```python
from build123d import *

# Parameters (mm, degrees)
F1_DEPTH  = 25
F2_W      = 2.8
F2_H      = 0.75
F3_DEPTH  = 1.5
F4_W      = 3.6
F4_H      = 1
F5_DEPTH  = 0.5
F6_W      = 10
F6_H      = 0.25
F7_DEPTH  = 0.2
F8_W      = 10
F8_H      = 14.625
F9_DEPTH  = 4.201
F10_R     = 1
F12_DEPTH = 2.701


with BuildPart() as f1:
    # F0 (on Front) → F1 (new body, symmetric)
    with BuildSketch(Plane.XZ):
        Polygon((-5, 4.2), (-5, 0), (5, 0), (5, 4.2), (1.4, 4.2), (1.4, 2), (-1.4, 2), (-1.4, 4.2), align=None)
    extrude(amount=F1_DEPTH, both=True)

    # F2 (on face) → F3 (join)
    with BuildSketch(Plane.XY.offset(2)):
        Rectangle(F2_W, F2_H)
    extrude(amount=F3_DEPTH)

    # F4 (on face) → F5 (join)
    with BuildSketch(Plane.XY.offset(4.2)):
        with Locations((3.2, -0.875)):
            Rectangle(F4_W, F4_H)
        with Locations((-3.2, -0.875)):
            Rectangle(F4_W, F4_H)
    extrude(amount=F5_DEPTH)

    # F6 (on face) → F7 (cut)
    with BuildSketch(Plane.XY.offset(4.2)):
        with Locations((0, -6.375)):
            Rectangle(F6_W, F6_H)
        with Locations((0, -11.375)):
            Rectangle(F6_W, F6_H)
        with Locations((0, -16.375)):
            Rectangle(F6_W, F6_H)
    extrude(amount=-F7_DEPTH, mode=Mode.SUBTRACT)

    # F8 (on face) → F9 (cut, through all)
    with BuildSketch(Plane.XY.offset(4.2)):
        with Locations((0, 17.6875)):
            Rectangle(F8_W, F8_H)
    extrude(amount=-F9_DEPTH, mode=Mode.SUBTRACT)

    # F10
    f10_edges = [f1.edges().sort_by_distance(p)[0] for p in [
        (-5, 10.375, 2.1),
        (5, 10.375, 2.1),
        (-5, -25, 2.1),
        (5, -25, 2.1),
    ]]
    fillet(f10_edges, radius=F10_R)

    # F11 (on face) → F12 (cut, through all)
    with BuildSketch(Plane.XY.offset(2)):
        Polygon((2, -0.375), (-2, -0.375), (-1.4, -3.375), (1.4, -3.375), align=None)
        Polygon((-1.4, 3.375), (-2, 0.375), (2, 0.375), (1.4, 3.375), align=None)
    extrude(amount=F12_DEPTH, mode=Mode.SUBTRACT)


solid = f1.part
```
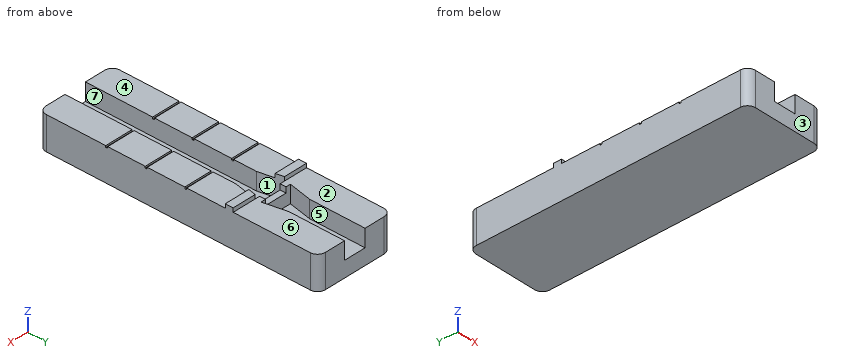
Read the model definition and answer for the solid it produces. Units are mm, in the model's axes. Face numbers are marked on the shaded views. A direction names the side the tool comes from. Coordinates: 2 decimals unless noted, no trailing zeros. Write each loop counter-clockwise with the first axis right and the second up, starting at its lowest first coordinate (ties: lowest second). Pieces come first, ordered by that corner, then holes. Notation, with made-up numbers: (-27.75, 20.25) -> (25.25, 20.25) arc R28 ccw to (25.25, 51.25) -> close; hole circle Ø1 at (56, 52.5). An arc over 180 degrees is marked (long way). Return JSON: item names as keys, results as strings.
1. Each of these flat-tipped pins is pushed along its axis until it touches: P1, Ø4, axis at x = 4, y = -4.5, coming from the +Z side; P2, Ø3, axis at x = -4, y = -2.5, coming from the +Z side. Where does it stop, or does it pass through?
Found:
{"P1": "z = 4.2", "P2": "z = 4.7"}
2. A cutting plane is placed at D-D (x = -2.75). Determine the outline of the cut face in (y, z) (3 decimals), and give its area (3 significant figures).
Found:
{"outline": "(-25, 0) -> (10.375, 0) -> (10.375, 4.2) -> (-0.375, 4.2) -> (-0.375, 4.7) -> (-1.375, 4.7) -> (-1.375, 4.2) -> (-6.25, 4.2) -> (-6.25, 4) -> (-6.5, 4) -> (-6.5, 4.2) -> (-11.25, 4.2) -> (-11.25, 4) -> (-11.5, 4) -> (-11.5, 4.2) -> (-16.25, 4.2) -> (-16.25, 4) -> (-16.5, 4) -> (-16.5, 4.2) -> (-25, 4.2) -> close", "area": "149 mm2"}
3. Find the intervals of material crossed by line 1 along X through (y, z) = (-22, 2.6); line 2 along Z through (x, y) = (-2.75, -23); line 3 along Z through (x, y) = (-1.25, -13), in increasing order. Write a range as from..to.
Found:
{"line 1": "-5..-1.4, 1.4..5", "line 2": "0..4.2", "line 3": "0..2"}
4. A cutting plane is placed at A-A (y = -15). Determine the outline of the cut face in (x, z), and give its area (3 significant figures).
Found:
{"outline": "(-5, 0) -> (5, 0) -> (5, 4.2) -> (1.4, 4.2) -> (1.4, 2) -> (-1.4, 2) -> (-1.4, 4.2) -> (-5, 4.2) -> close", "area": "35.8 mm2"}
5. A tool of negligible diameter and unlimited length cuts with its end or side. For the marked faces 4, 5, 6 and 7, from which of +Z, -Z, +X, -X, +Y, -Y can it reach the whole face along a straight path? Write none if from no direction.
Found:
{"face 4": "+Z, +X, -X, -Y", "face 5": "+Z, +Y", "face 6": "+Z, +X, -X, +Y", "face 7": "+Z, -Y"}
6. A cutting plane is placed at C-C (z = 3.15). Determine the outline of the cut face in (x, y) (3 decimals), and give its area (3 significant figures).
Found:
{"outline": "(-5, -24) arc R1 ccw to (-4, -25) -> (-1.4, -25) -> (-1.4, -3.375) -> (-2, -0.375) -> (2, -0.375) -> (1.4, -3.375) -> (1.4, -25) -> (4, -25) arc R1 ccw to (5, -24) -> (5, 9.375) arc R1 ccw to (4, 10.375) -> (1.4, 10.375) -> (1.4, 3.375) -> (2, 0.375) -> (-2, 0.375) -> (-1.4, 3.375) -> (-1.4, 10.375) -> (-4, 10.375) arc R1 ccw to (-5, 9.375) -> close", "area": "252 mm2"}
7. A cutting plane is placed at B-B (x = 0). Determine the outline of the cut face in (y, z) (3 decimals), and give its area (3 significant figures).
Found:
{"outline": "(-25, 0) -> (10.375, 0) -> (10.375, 2) -> (0.375, 2) -> (0.375, 3.5) -> (-0.375, 3.5) -> (-0.375, 2) -> (-25, 2) -> close", "area": "71.9 mm2"}
8. Determine the mould class of the marked faces 1, 2 and 3 for opening direction Y: pulls with the +Y half, pulls with the -Y half, needs draft (parallel to the pull), parting line crosses it, or undercut.
Found:
{"face 1": "undercut", "face 2": "needs draft", "face 3": "pulls with the -Y half"}
